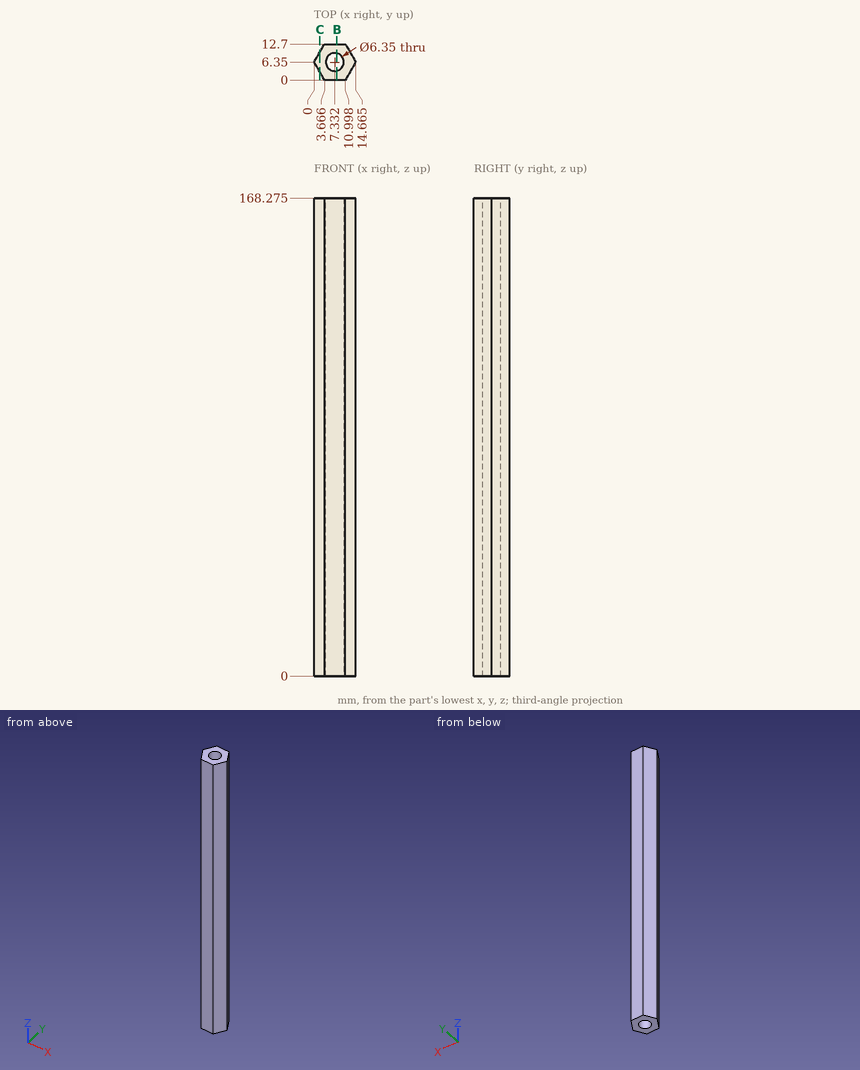
Can you work these out from the drawing? Everything is in mm from the part's minimum corner. Give positions to 0.01 mm unless a question says otherwise; leave off trailing zeros. Order: outer loops, then holes, each group sorted by start corner. A loop starts at its lowest first (then second) coordinate and runs counter-clockwise, first axis right, second up. Notation, with made-up numbers: M 40.25,-25 L 74.25,-25 A22 cw 74.25,10 Z; hole C 2,50 d7. An arc over 180 degrees is marked long. One line per item, written item: value.
Item 1: Please list where these lines run through material, in increasing order: line 1 (Y direction, x = 7, z = 121.5); line 2 (Y direction, x = 6.5, z = 98) (1 decimal); line 3 (X direction, y = 5.25, z = 90) (1 decimal).
Verdict:
line 1: 0 to 3.19, 9.51 to 12.7
line 2: 0 to 3.3, 9.4 to 12.7
line 3: 0.6 to 4.4, 10.3 to 14
Item 2: If we section it at B-B on x = 8: Write out the boundary of the cut face in (y, z) (1 decimal).
Verdict:
outline: M 0,0 L 3.2,0 L 3.2,168.3 L 0,168.3 Z; M 9.5,0 L 12.7,0 L 12.7,168.3 L 9.5,168.3 Z
Item 3: If we section it at C-C on x = 2: Write out the boundary of the cut face in (y, z) (1 decimal), and give its area (3 significant figures).
Verdict:
outline: M 2.9,0 L 9.8,0 L 9.8,168.3 L 2.9,168.3 Z
area: 1,170 mm2
Item 4: For pin 1 (5.5 mm diameter, centred on x = 7.33, y = 6.35, fed in from -Z), with a flat end and sliding along its axis, tell me the tip position at first contact or that it passes through.
Verdict:
pin 1: through
